from build123d import *

# Parameters (mm, degrees)
BOSS_EXTRUDE1_DEPTH = 15.4
BOSS_EXTRUDE2_DEPTH = 5
SCALE_1_SCALE       = 2.5


with BuildPart() as part:
    # Sketch1 → Boss-Extrude1 (new body)
    with BuildSketch(Plane(origin=(0, -3, 0), x_dir=(1, 0, 0), z_dir=(0, 1, 0))):
        with BuildLine():
            Line((-51.8, -4), (-49.76, -4))
            Line((-49.76, -4), (-48.626761605, -4.978453238))
            ThreePointArc((-48.626761605, -4.978453238), (-48.302157504, -5.099995345), (-47.97651659, -4.981259077))
            Line((-47.97651659, -4.981259077), (-46.82, -4))
            Line((-46.82, -4), (-46.641421356, -4))
            Line((-46.641421356, -4), (-46.5, -3.858578644))
            Line((-46.5, -3.858578644), (-46.5, 3.858578644))
            Line((-46.5, 3.858578644), (-46.641421356, 4))
            Line((-46.641421356, 4), (-46.82, 4))
            Line((-46.82, 4), (-47.996771021, 4.897557777))
            ThreePointArc((-47.996771021, 4.897557777), (-48.302073982, 4.999995699), (-48.606516627, 4.895028552))
            Line((-48.606516627, 4.895028552), (-49.76, 4))
            Line((-49.76, 4), (-51.8, 4))
            Line((-51.8, 4), (-51.8, -4))
        make_face()
    extrude(amount=-BOSS_EXTRUDE1_DEPTH)

    # Sketch2 → Boss-Extrude2 (add)
    with BuildSketch(Plane(origin=(0, -10.45, 0), x_dir=(1, 0, 0), z_dir=(0, 1, 0))):
        Polygon((-67.5, 3.858578644), (-67.5, -3.858578644), (-67.358578644, -4), (-51.8, -4), (-51.8, 4), (-67.358578644, 4), align=None)
    extrude(amount=-BOSS_EXTRUDE2_DEPTH)

    # Sketch3 → Cut-Revolve1 (revolve, cut)
    with BuildSketch(Plane.XY, mode=Mode.PRIVATE) as cut_revolve1_sk:
        Polygon((-63.5, -15.45), (-65, -15.45), (-64.7295, -15.1795), (-64.7295, -10.7105), (-65, -10.44), (-63.5, -10.44), align=None)
    revolve(cut_revolve1_sk.sketch.rotate(Axis((-63.5, -10.44, 0), (0, -1, 0)), 90), axis=Axis((-63.5, -10.44, 0), (0, -1, 0)), mode=Mode.SUBTRACT)

    # Sketch4 → Cut-Revolve2 (revolve, cut)
    with BuildSketch(Plane.XY, mode=Mode.PRIVATE) as cut_revolve2_sk:
        Polygon((-56.5, -15.45), (-58, -15.45), (-57.7295, -15.1795), (-57.7295, -10.7105), (-58, -10.44), (-56.5, -10.44), align=None)
    revolve(cut_revolve2_sk.sketch.rotate(Axis((-56.5, -10.44, 0), (0, -1, 0)), 90), axis=Axis((-56.5, -10.44, 0), (0, -1, 0)), mode=Mode.SUBTRACT)


with BuildPart() as part_1:
    # Scale 1: scaled about (-53.834630524, -11.714177537, 0.010190259)
    add(part.part.scale(SCALE_1_SCALE).moved(Location((80.751945786, 17.571266306, -0.015285389))))


solid = part_1.part
Build history of the part. All positions in model axes, mm. A direction names the side the tool comes from. Round coordinates to 2 decimals unless told otherwise and drop trailing zeros. Write each loop counter-clockwise with the first axis right and the second up, starting at its lowest first coordinate (ties: lowest second). Pieces come first, ordered by that corner, then holes. Notation, with made-up numbers: (26.25, 57) - (68.25, 57) arc R13 cw to (68.25, 80) - close; hole circle Ø6 at (-11, -27.75). An arc over 180 degrees is marked (long way). One line per question, with ' | ' between items.
1. Drill centre lines: line 1 along Y through (x, z) = (-50, -6); line 2 along Z through (x, y) = (-73.5, -14); line 3 along X through (y, z) = (-4, 5.5). Where is each one in solid material? Low to high. Write a range as from..to.
Results are:
line 1: -21.05..-8.55 | line 2: -10.02..9.98 | line 3: -48.75..-35.5
2. Band-saw the part on D-D, the plane z = 1. Give the number of separate pieces and of enclosed holes in the cut face, and give its area (3 significant figures).
Results are:
separate pieces: 3 | enclosed holes: 0 | area: 854 mm^2
3. Mould opens along Z. For faces 4 (the face through (-37.748, -8.909, -11.122)), 5 (the face through (-79.9, -14.7, 2.4)), 6 (the face through (-69, -8.554, 0)) say: released by +Z, released by -Z, zero draft, split by the parting line, or undercut.
Results are:
face 4: released by -Z | face 5: undercut | face 6: zero draft
4. Tool access for faces 1 (the face through (-69, -21.054, 0)), 2 (the face through (-60, -13, -10.015)), 3 (the face through (-48.748, 1, 0)): list every direction of +Z, -Z, +X, -X, +Y, -Y with a clear straight run to the whole face (end or side of a thin tool).
Results are:
face 1: +Z, -Z, -X, -Y | face 2: -Z, -X, +Y, -Y | face 3: +Z, -Z, -X, +Y
5. Drop flat-ended pins along their axis: pin 1 Ø2 at (y, z) = (-23.5, 3.5) entering from -X; pin 2 Ø1.5 at (x, y) = (-62.5, -16) entering from +Z; pin 3 Ø8 at (x, z) = (-60.5, -0.02) entering from -Y. Give the stop position or say it passes through.
Results are:
pin 1: x = -48.75 | pin 2: z = 9.98 | pin 3: y = -21.05
6. Band-saw the part on B-B, the plane z = -4.5. Write the cut outline in (x, y), and give its area (3 significant figures).
Results are:
outline: (-88, -21.05) - (-48.75, -21.05) - (-48.75, -28.43) - (-35.5, -28.43) - (-35.5, 10.07) - (-48.75, 10.07) - (-48.75, -8.55) - (-88, -8.55) - close | area: 1,000 mm^2
7. Band-saw the part on C-C, the plane x = -50. Write the cut outline in (y, z).
Results are:
outline: (-21.05, -10.02) - (-8.55, -10.02) - (-8.55, 9.98) - (-21.05, 9.98) - close
8. Band-saw the part on A-A, the plane y = -23.5. Write the cut outline in (x, z), and give its area (3 significant figures).
Results are:
outline: (-48.75, -10.02) - (-43.65, -10.02) - (-40.76, -12.25) arc R1.25 ccw to (-39.24, -12.26) - (-36.3, -10.02) - (-35.85, -10.02) - (-35.5, -9.66) - (-35.5, 9.63) - (-35.85, 9.98) - (-36.3, 9.98) - (-39.19, 12.44) arc R1.25 ccw to (-40.81, 12.43) - (-43.65, 9.98) - (-48.75, 9.98) - close | area: 286 mm^2
